Can you work these out from the model? Positions are in its coordinate system, mm. Face numbers are marked on the shaded views. Round coordinates to 2 decimals unless told otherwise and drop trailing zeros. Loops run counter-clockwise (first coordinate to the right, second up) from the corner with the lowest first, then second, coordinate; pieces in that order, holes last.
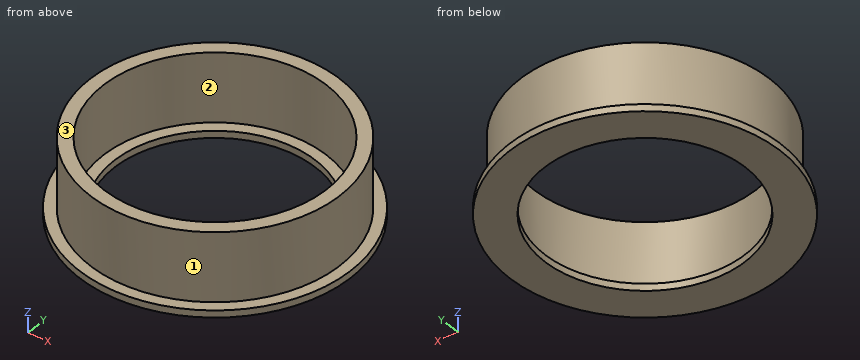
from build123d import *

# Parameters (mm, degrees)
F0_R     = 33.734375
F1_DEPTH = 1.75
F2_R     = 31.05
F2_R_2   = 27.75
F3_DEPTH = 17.15
F2_R_3   = 25
F4_DEPTH = 1.751


with BuildPart() as f1:
    # F0 (on Top) → F1 (new body)
    with BuildSketch(Plane.XY):
        Circle(F0_R)
    extrude(amount=F1_DEPTH)

    # F2 (on face) → F3 (join)
    with BuildSketch(Plane.XY.offset(1.75)):
        Circle(F2_R)
        Circle(F2_R_2, mode=Mode.SUBTRACT)
    extrude(amount=F3_DEPTH)

    # F2 (on face) → F4 (cut, through all)
    with BuildSketch(Plane.XY.offset(1.75)):
        Circle(F2_R_3)
    extrude(amount=-F4_DEPTH, mode=Mode.SUBTRACT)


solid = f1.part
(1) If we section it at A-A, the plane y = 0: List the corners of the cut face in (x, z) for me, then the cut area to 3 significant figures.
Worked answers:
outline: (-33.73, 0) - (-25, 0) - (-25, 1.75) - (-27.75, 1.75) - (-27.75, 18.9) - (-31.05, 18.9) - (-31.05, 1.75) - (-33.73, 1.75) - close; (25, 0) - (33.73, 0) - (33.73, 1.75) - (31.05, 1.75) - (31.05, 18.9) - (27.75, 18.9) - (27.75, 1.75) - (25, 1.75) - close
area: 144 mm2
(2) Will these pins go through, and if not, where does the flat tip stop? P1, Ø6, axis at y = -18, z = 4, coming from the -X side; P2, Ø4, axis at y = 13, z = 2, coming from the -X side; P3, Ø4, axis at x = 27, z = 9.5, coming from the +Y side.
Worked answers:
P1: stops at x = -29.69
P2: stops at x = -31.89
P3: stops at y = 18.41
(3) If we mould it in two halves opening along X, with no side actions, what happens to the marked faces 1, 2 and 3? For each: released by +X, released by -X, zero draft, split by the parting line, or undercut.
Worked answers:
face 1: split by the parting line
face 2: undercut
face 3: zero draft
(4) If I drill on line 1 (Y direction, x = 0, z = 15.25); line 2 (Y direction, x = 21, z = 18); line 3 (Z direction, x = 1, y = 26), over which ranges is the centre line in solid material (lowest first)?
Worked answers:
line 1: y = -31.05 to -27.75, 27.75 to 31.05
line 2: y = -22.87 to -18.14, 18.14 to 22.87
line 3: z = 0 to 1.75
(5) If we section it at C-C, the plane z = 9: List the corners of the cut face in (x, y) for me.
Worked answers:
outline: circle Ø62.1 at (0, 0); hole circle Ø55.5 at (0, 0)
